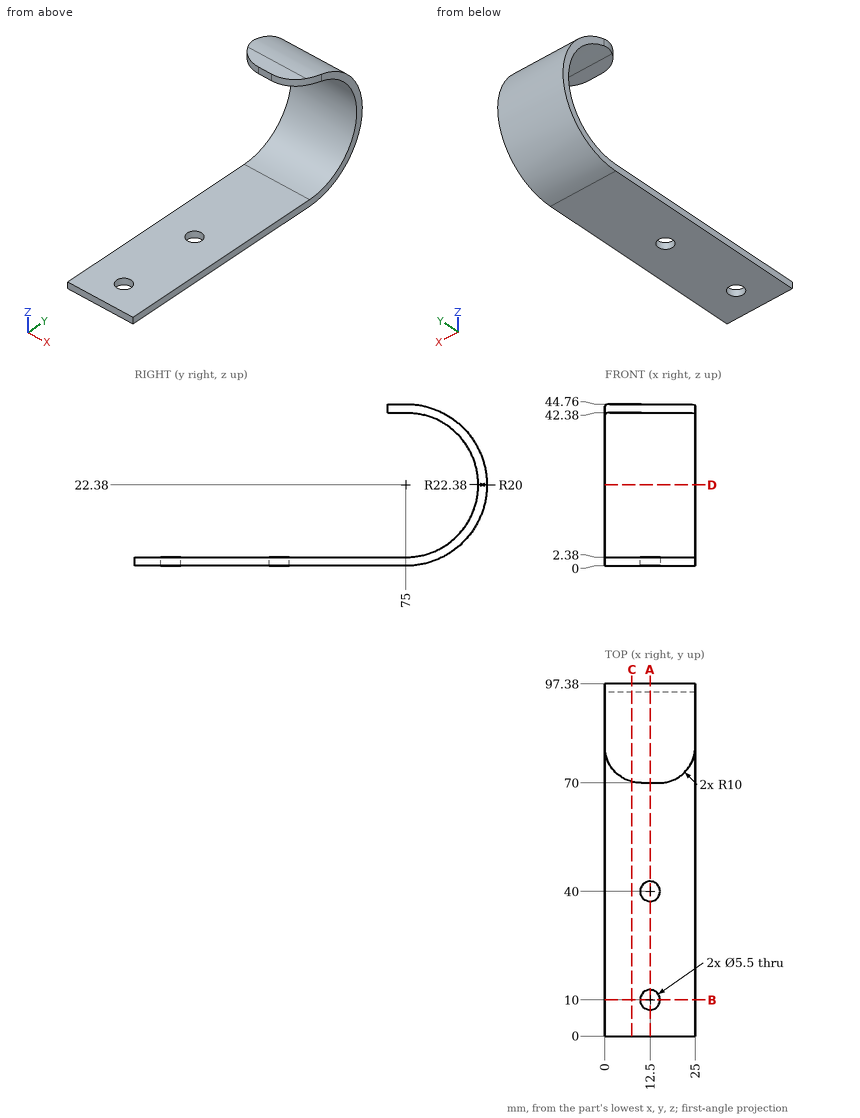
Study the drawing (mm; zero at the part's minimum x, y, z) and answer. Round coordinates to 2 decimals unless told otherwise and drop trailing zeros. Write each loop counter-clockwise with the first axis right and the second up, starting at its lowest first coordinate (ties: lowest second). Pieces come first, ordered by that corner, then holes. Notation, with made-up numbers: (58.5, 46.25) - (79.5, 46.25) arc R8 cw to (79.5, 55.25) - close; hole circle Ø8 at (54.5, 20). An arc over 180 degrees is marked (long way). Use a Markdown table: item, result. Add a question column.
1. The part is cut by section A-A (x = 12.5). Write down the section's boundary in (y, z).
2. Flat-ended cylindrical pins translate along their axes: P1, Ø6, axis at x = 13, z = 22.5, coming from the -Y side; P2, Ø3.5, axis at x = 12.5, y = 10, coming from the -Z side; P3, Ø1, axis at x = 13, y = 45, coming from the +Z side; P4, Ø10, axis at x = 20, z = 31, coming from the +Y side. Find the tip coordinate at first contact, or state that the pin passes through.
3. Consider line 1 (Y direction, x = 12.5, z = 1.7); line 2 (Z direction, x = 6.5, y = 30.5); line 3 (Y direction, x = 12.5, z = 1.9). Determine where each line is inside the solid, lowest interval first.
4. The part is cut by section D-D (z = 22.38). Write down the section's boundary in (x, y), and give its area (3 significant figures).
5. The part is cut by section B-B (y = 10). Write down the section's boundary in (x, z).
6. The part is cut by section C-C (x = 7.5). Write down the section's boundary in (y, z).
Reported:
| question | item | result |
|---|---|---|
| 1 | outline | (0, 0) - (7.25, 0) - (7.25, 2.38) - (0, 2.38) - close; (12.75, 0) - (37.25, 0) - (37.25, 2.38) - (12.75, 2.38) - close; (42.75, 0) - (75, 0) arc R22.38 ccw to (75, 44.76) - (70, 44.76) - (70, 42.38) - (75, 42.38) arc R20 cw to (75, 2.38) - (42.75, 2.38) - close |
| 2 | P1 | y = 94.76 |
| 2 | P2 | through |
| 2 | P3 | z = 2.38 |
| 2 | P4 | y = 97.09 |
| 3 | line 1 | 0 to 7.25, 12.75 to 37.25, 42.75 to 83.56 |
| 3 | line 2 | 0 to 2.38 |
| 3 | line 3 | 0 to 7.25, 12.75 to 37.25, 42.75 to 84.02 |
| 4 | outline | (0, 95) - (25, 95) - (25, 97.38) - (0, 97.38) - close |
| 4 | area | 59.5 mm^2 |
| 5 | outline | (0, 0) - (9.75, 0) - (9.75, 2.38) - (0, 2.38) - close; (15.25, 0) - (25, 0) - (25, 2.38) - (15.25, 2.38) - close |
| 6 | outline | (0, 0) - (75, 0) arc R22.38 ccw to (75, 44.76) - (70.32, 44.76) - (70.32, 42.38) - (75, 42.38) arc R20 cw to (75, 2.38) - (0, 2.38) - close |
